Geometry: final body of the model. Coordinates: model frame, mm. A direction names the side the tool comes from. Give positions to 0.01 mm unless a question says otherwise; leave off trailing zeros. Write each loop counter-clockwise with the first axis right and the second up, starting at its lowest first coordinate (ties: lowest second). Pieces come first, ordered by that corner, then holes. Notation, with made-up numbers: (21.25, -28) - (56.25, -28) arc R21 ccw to (56.25, 5) - close; hole circle Ø4 at (-39.5, 81). An arc over 180 degrees is marked (long way). One line per question, with ' | ' between items. Start each with the question number.
```python
from build123d import *

# Parameters (mm, degrees)
SKETCH_2_W          = 150
SKETCH_2_H          = 140
EXTRUDE_1_DEPTH     = 140
SKETCH_3_W          = 150
SKETCH_3_H          = 100
CUT_EXTRUDE_1_DEPTH = 110
SKETCH_4_W          = 100
SKETCH_4_H          = 13
CUT_EXTRUDE_2_DEPTH = 231.131739112
SKETCH_5_R          = 3
CUT_EXTRUDE_3_DEPTH = 50
SKETCH_6_R          = 3
CUT_EXTRUDE_4_DEPTH = 177.679477459
SKETCH_7_R          = 20
SKETCH_7_R_2        = 10
EXTRUDE_1_2_DEPTH   = 10
SKETCH_8_W          = 10
SKETCH_8_H          = 10
CUT_EXTRUDE_5_DEPTH = 120
SKETCH_10_W         = 20
SKETCH_10_H         = 5
CUT_EXTRUDE_7_DEPTH = 120
EXTRUDE_2_DEPTH     = 10


with BuildPart() as part:
    # 草圖2 → Extrude 1 (new body)
    with BuildSketch(Plane(origin=(0, 0, 0), x_dir=(1, 0, 0), z_dir=(0, 1, 0))):
        with Locations((15.857142857, -34.214285714)):
            Rectangle(SKETCH_2_W, SKETCH_2_H)
    extrude(amount=EXTRUDE_1_DEPTH)

    # 草圖3 → 除料-伸長1 (cut)
    with BuildSketch(Plane(origin=(0, 140, 0), x_dir=(1, 0, 0), z_dir=(0, 1, 0))):
        with Locations((15.857142857, -34.214285714)):
            Rectangle(SKETCH_3_W, SKETCH_3_H)
    extrude(amount=-CUT_EXTRUDE_1_DEPTH, mode=Mode.SUBTRACT)

    # 草圖4 → 除料-伸長2 (cut, through all)
    with BuildSketch(Plane(origin=(90.857142857, 0, 0), x_dir=(0, 0, -1), z_dir=(1, 0, 0))):
        with Locations((-34.214285714, 13.5)):
            Rectangle(SKETCH_4_W, SKETCH_4_H)
    extrude(amount=-CUT_EXTRUDE_2_DEPTH, mode=Mode.SUBTRACT)

    # 草圖5 → 除料-伸長3 (cut)
    with BuildSketch(Plane(origin=(0, 30, 0), x_dir=(1, 0, 0), z_dir=(0, 1, 0))):
        with Locations(Location((70.857142857, -34.214285714, 0), (0, 0, 270))):
            Circle(SKETCH_5_R)
    extrude(amount=-CUT_EXTRUDE_3_DEPTH, mode=Mode.SUBTRACT)

    # 草圖6 → 除料-伸長4 (cut, through all)
    with BuildSketch(Plane(origin=(0, 30, 0), x_dir=(1, 0, 0), z_dir=(0, 1, 0))):
        with Locations(Location((-29.142857143, -34.214285714, 0), (0, 0, 270))):
            Circle(SKETCH_6_R)
    extrude(amount=-CUT_EXTRUDE_4_DEPTH, mode=Mode.SUBTRACT)

    # 草圖7 → Extrude 1 2 (add)
    with BuildSketch(Plane(origin=(0, 140, 0), x_dir=(1, 0, 0), z_dir=(0, 1, 0))):
        with Locations((15.857142857, -114.214285714)):
            Circle(SKETCH_7_R)
        with Locations((15.857142857, -114.214285714)):
            Circle(SKETCH_7_R_2, mode=Mode.SUBTRACT)
    extrude(amount=-EXTRUDE_1_2_DEPTH)

    # 草圖8 → 除料-伸長5 (cut)
    with BuildSketch(Plane(origin=(0, 140, 0), x_dir=(1, 0, 0), z_dir=(0, 1, 0))):
        with Locations((16.382857537, 30.785714286)):
            Rectangle(SKETCH_8_W, SKETCH_8_H)
    extrude(amount=-CUT_EXTRUDE_5_DEPTH, mode=Mode.SUBTRACT)

    # 草圖10 → 除料-伸長7 (cut)
    with BuildSketch(Plane(origin=(0, 140, 0), x_dir=(1, 0, 0), z_dir=(0, 1, 0))):
        with Locations((16.382857537, 28.285714286)):
            Rectangle(SKETCH_10_W, SKETCH_10_H)
    extrude(amount=-CUT_EXTRUDE_7_DEPTH, mode=Mode.SUBTRACT)

    # 草圖11 → 填料-伸長2 (add)
    with BuildSketch(Plane.XY.offset(104.214285714)):
        with BuildLine():
            Line((-59.142857143, 82.136050004), (-59.142857143, 0))
            Line((-59.142857143, 0), (90.857142857, 0))
            Line((90.857142857, 0), (90.857142857, 59.85891712))
            add(Edge.make_bspline(
                [(-59.142857143, 82.136050004), (-2.260684415, 0.574504188), (33.520042851, 85.660046613), (90.857142857, 59.85891712)],
                knots=[0, 0, 0, 0, 1, 1, 1, 1], degree=3))
        make_face()
    extrude(amount=EXTRUDE_2_DEPTH)


solid = part.part
```
1) Section C-C, the plane z = 120.5. Output: boundary loops of the cut face in (x, y).
2) Section A-A, the plane y = 126. Output: boundary loops of the cut face in (x, z), plus the area to 3 significant figures.
3) Line query: L1, parallel to Y at x = 22, z = 23; L2, parallel to Z at x = -6.5, y = 109; L3, parallel to Z at x = 9, y = 106.5. Output: solid intervals per line, ascending.
4) Section B-B, the plane z = 49.5. Output: boundary loops of the cut face in (x, y).
5) First-contact query: pin 1 Ø1.5 at (x, y) = (25, 87) entering from +Z; pin 2 Ø8 at (x, z) = (70.86, 34.21) entering from +Y. Flat tips, straight axial feed; report the tip coordinate or a pass-through.
6) Pull-direction query (Z, two-part tool) for faces 6 (the flat face through (26.383, 81, -28)), 7 (the flat face through (90.857, 22, 38)); classes: +Z half, -Z half, draft (parallel to the pull), parting line (faces both ways), or undercut.
7) Reachability of faces 1 (the flat face through (9, 81, -30.786)), 2 (the cylindrical face through (71.758, 3.549, 37.076)), 3 (the flat face through (21.383, 81, -33)), 4 (the flat face through (17, 13, 84.214)), 5 (the flat face through (15, 30, 34)) from +Z, -Z, +X, -X, +Y, -Y: full face, straight path, thin tool, end or side. Return the list, or none.
Answer key:
1) outline: (-3.13, 130) - (8.08, 130) - (8.08, 140) - (-3.13, 140) - close; (23.63, 130) - (34.84, 130) - (34.84, 140) - (23.63, 140) - close
2) outline: (-59.14, -35.79) - (11.38, -35.79) - (11.38, -30.79) - (6.38, -30.79) - (6.38, -25.79) - (26.38, -25.79) - (26.38, -30.79) - (21.38, -30.79) - (21.38, -35.79) - (90.86, -35.79) - (90.86, -15.79) - (-59.14, -15.79) - close; (-59.14, 84.21) - (90.86, 84.21) - (90.86, 104.21) - (-59.14, 104.21) - close | area: 5,850 mm^2
3) L1: 0 to 7, 20 to 30 | L2: -35.79 to -15.79, 84.21 to 104.21 | L3: -35.79 to -30.79, -25.79 to -15.79, 84.21 to 104.21
4) outline: (-59.14, 0) - (90.86, 0) - (90.86, 7) - (-59.14, 7) - close; (-59.14, 20) - (90.86, 20) - (90.86, 30) - (-59.14, 30) - close
5) pin 1: z = 104.21 | pin 2: y = 30
6) face 6: undercut | face 7: draft
7) face 1: +Y | face 2: +Y, -Y | face 3: -Z, +Y | face 4: +X, -X | face 5: +X, -X, +Y
